from build123d import *

# Parameters (mm, degrees)
F0_R     = 2.7686
F1_DEPTH = 13.208
F2_DEPTH = 10.922
F3_DEPTH = 0.254
F4_DEPTH = 4.953
F5_R     = 2.7686
F6_DEPTH = 6.731
F7_DEPTH = 0.381


with BuildPart() as f1:
    # F0 (on Top) → F1 (new body)
    with BuildSketch(Plane.XY):
        with BuildLine():
            Line((-13.6779, -4.1021), (13.6779, -4.1021))
            ThreePointArc((13.6779, -4.1021), (17.78, 0), (13.6779, 4.1021))
            Line((13.6779, 4.1021), (-13.6779, 4.1021))
            ThreePointArc((-13.6779, 4.1021), (-17.78, 0), (-13.6779, -4.1021))
        make_face()
        with BuildLine():
            ThreePointArc((-13.6779, -3.7211), (-17.399, 0), (-13.6779, 3.7211))
            Line((-13.6779, 3.7211), (13.6779, 3.7211))
            ThreePointArc((13.6779, 3.7211), (17.399, 0), (13.6779, -3.7211))
            Line((13.6779, -3.7211), (-13.6779, -3.7211))
        make_face(mode=Mode.SUBTRACT)
        with BuildLine():
            Line((13.6779, 3.7211), (-13.6779, 3.7211))
            ThreePointArc((-13.6779, 3.7211), (-17.399, 0), (-13.6779, -3.7211))
            Line((-13.6779, -3.7211), (13.6779, -3.7211))
            ThreePointArc((13.6779, -3.7211), (17.399, 0), (13.6779, 3.7211))
        make_face()
        with BuildLine():
            ThreePointArc((-12.875422, 0.0127), (-12.875422, 2.4003), (-10.8077, 3.5941))
            Line((-10.8077, 3.5941), (10.8077, 3.5941))
            ThreePointArc((10.8077, 3.5941), (12.875422, 2.4003), (12.875422, 0.0127))
            Line((12.875422, 0.0127), (11.482276, -2.4003))
            ThreePointArc((11.482276, -2.4003), (10.608354, -3.274222), (9.414554, -3.5941))
            Line((9.414554, -3.5941), (-9.414554, -3.5941))
            ThreePointArc((-9.414554, -3.5941), (-10.608354, -3.274222), (-11.482276, -2.4003))
            Line((-11.482276, -2.4003), (-12.875422, 0.0127))
        make_face(mode=Mode.SUBTRACT)
        with BuildLine():
            Line((10.8077, 3.5941), (-10.8077, 3.5941))
            ThreePointArc((-10.8077, 3.5941), (-12.875422, 2.4003), (-12.875422, 0.0127))
            Line((-12.875422, 0.0127), (-11.482276, -2.4003))
            ThreePointArc((-11.482276, -2.4003), (-10.608354, -3.274222), (-9.414554, -3.5941))
            Line((-9.414554, -3.5941), (9.414554, -3.5941))
            ThreePointArc((9.414554, -3.5941), (10.608354, -3.274222), (11.482276, -2.4003))
            Line((11.482276, -2.4003), (12.875422, 0.0127))
            ThreePointArc((12.875422, 0.0127), (12.875422, 2.4003), (10.8077, 3.5941))
        make_face()
        with BuildLine():
            ThreePointArc((-12.325496, 0.3302), (-12.325496, 2.0828), (-10.8077, 2.9591))
            Line((-10.8077, 2.9591), (10.8077, 2.9591))
            ThreePointArc((10.8077, 2.9591), (12.325496, 2.0828), (12.325496, 0.3302))
            Line((12.325496, 0.3302), (10.93235, -2.0828))
            ThreePointArc((10.93235, -2.0828), (10.290854, -2.724296), (9.414554, -2.9591))
            Line((9.414554, -2.9591), (-9.414554, -2.9591))
            ThreePointArc((-9.414554, -2.9591), (-10.290854, -2.724296), (-10.93235, -2.0828))
            Line((-10.93235, -2.0828), (-12.325496, 0.3302))
        make_face(mode=Mode.SUBTRACT)
        with BuildLine():
            Line((10.8077, 2.9591), (-10.8077, 2.9591))
            ThreePointArc((-10.8077, 2.9591), (-12.325496, 2.0828), (-12.325496, 0.3302))
            Line((-12.325496, 0.3302), (-10.93235, -2.0828))
            ThreePointArc((-10.93235, -2.0828), (-10.290854, -2.724296), (-9.414554, -2.9591))
            Line((-9.414554, -2.9591), (9.414554, -2.9591))
            ThreePointArc((9.414554, -2.9591), (10.290854, -2.724296), (10.93235, -2.0828))
            Line((10.93235, -2.0828), (12.325496, 0.3302))
            ThreePointArc((12.325496, 0.3302), (12.325496, 2.0828), (10.8077, 2.9591))
        make_face()
        with Locations((-8.717981, 0)):
            Circle(F0_R, mode=Mode.SUBTRACT)
        with Locations((8.717981, 0)):
            Circle(F0_R, mode=Mode.SUBTRACT)
    extrude(amount=-F1_DEPTH)

    # F0 (on Top) → F2 (cut)
    with BuildSketch(Plane.XY):
        with BuildLine():
            Line((-13.6779, -4.1021), (13.6779, -4.1021))
            ThreePointArc((13.6779, -4.1021), (17.78, 0), (13.6779, 4.1021))
            Line((13.6779, 4.1021), (-13.6779, 4.1021))
            ThreePointArc((-13.6779, 4.1021), (-17.78, 0), (-13.6779, -4.1021))
        make_face()
        with BuildLine():
            ThreePointArc((-13.6779, -3.7211), (-17.399, 0), (-13.6779, 3.7211))
            Line((-13.6779, 3.7211), (13.6779, 3.7211))
            ThreePointArc((13.6779, 3.7211), (17.399, 0), (13.6779, -3.7211))
            Line((13.6779, -3.7211), (-13.6779, -3.7211))
        make_face(mode=Mode.SUBTRACT)
    extrude(amount=-F2_DEPTH, mode=Mode.SUBTRACT)

    # F0 (on Top) → F3 (cut)
    with BuildSketch(Plane.XY):
        with BuildLine():
            Line((13.6779, 3.7211), (-13.6779, 3.7211))
            ThreePointArc((-13.6779, 3.7211), (-17.399, 0), (-13.6779, -3.7211))
            Line((-13.6779, -3.7211), (13.6779, -3.7211))
            ThreePointArc((13.6779, -3.7211), (17.399, 0), (13.6779, 3.7211))
        make_face()
        with BuildLine():
            ThreePointArc((-12.875422, 0.0127), (-12.875422, 2.4003), (-10.8077, 3.5941))
            Line((-10.8077, 3.5941), (10.8077, 3.5941))
            ThreePointArc((10.8077, 3.5941), (12.875422, 2.4003), (12.875422, 0.0127))
            Line((12.875422, 0.0127), (11.482276, -2.4003))
            ThreePointArc((11.482276, -2.4003), (10.608354, -3.274222), (9.414554, -3.5941))
            Line((9.414554, -3.5941), (-9.414554, -3.5941))
            ThreePointArc((-9.414554, -3.5941), (-10.608354, -3.274222), (-11.482276, -2.4003))
            Line((-11.482276, -2.4003), (-12.875422, 0.0127))
        make_face(mode=Mode.SUBTRACT)
    extrude(amount=-F3_DEPTH, mode=Mode.SUBTRACT)

    # F0 (on Top) → F4 (cut)
    with BuildSketch(Plane.XY):
        with BuildLine():
            Line((10.8077, 2.9591), (-10.8077, 2.9591))
            ThreePointArc((-10.8077, 2.9591), (-12.325496, 2.0828), (-12.325496, 0.3302))
            Line((-12.325496, 0.3302), (-10.93235, -2.0828))
            ThreePointArc((-10.93235, -2.0828), (-10.290854, -2.724296), (-9.414554, -2.9591))
            Line((-9.414554, -2.9591), (9.414554, -2.9591))
            ThreePointArc((9.414554, -2.9591), (10.290854, -2.724296), (10.93235, -2.0828))
            Line((10.93235, -2.0828), (12.325496, 0.3302))
            ThreePointArc((12.325496, 0.3302), (12.325496, 2.0828), (10.8077, 2.9591))
        make_face()
        with Locations((-8.717981, 0)):
            Circle(F0_R, mode=Mode.SUBTRACT)
        with Locations((8.717981, 0)):
            Circle(F0_R, mode=Mode.SUBTRACT)
    extrude(amount=-F4_DEPTH, mode=Mode.SUBTRACT)

    # F5 (on face) → F6 (cut)
    with BuildSketch(Plane(origin=(0, 0, -13.208), x_dir=(1, 0, 0), z_dir=(0, 0, -1))):
        with BuildLine():
            ThreePointArc((-12.325496, -0.3302), (-12.325496, -2.0828), (-10.8077, -2.9591))
            Line((-10.8077, -2.9591), (10.8077, -2.9591))
            ThreePointArc((10.8077, -2.9591), (12.325496, -2.0828), (12.325496, -0.3302))
            Line((12.325496, -0.3302), (10.93235, 2.0828))
            ThreePointArc((10.93235, 2.0828), (10.290854, 2.724296), (9.414554, 2.9591))
            Line((9.414554, 2.9591), (-9.414554, 2.9591))
            ThreePointArc((-9.414554, 2.9591), (-10.290854, 2.724296), (-10.93235, 2.0828))
            Line((-10.93235, 2.0828), (-12.325496, -0.3302))
        make_face()
        with Locations((-8.717981, 0)):
            Circle(F5_R, mode=Mode.SUBTRACT)
        with Locations((8.717981, 0)):
            Circle(F5_R, mode=Mode.SUBTRACT)
    extrude(amount=-F6_DEPTH, mode=Mode.SUBTRACT)

    # F5 (on face) → F7 (cut)
    with BuildSketch(Plane(origin=(0, 0, -13.208), x_dir=(1, 0, 0), z_dir=(0, 0, -1))):
        with BuildLine():
            ThreePointArc((13.6779, -3.7211), (17.399, 0), (13.6779, 3.7211))
            Line((13.6779, 3.7211), (-13.6779, 3.7211))
            ThreePointArc((-13.6779, 3.7211), (-17.399, 0), (-13.6779, -3.7211))
            Line((-13.6779, -3.7211), (13.6779, -3.7211))
        make_face()
        with BuildLine():
            Line((10.8077, -2.9591), (-10.8077, -2.9591))
            ThreePointArc((-10.8077, -2.9591), (-12.325496, -2.0828), (-12.325496, -0.3302))
            Line((-12.325496, -0.3302), (-10.93235, 2.0828))
            ThreePointArc((-10.93235, 2.0828), (-10.290854, 2.724296), (-9.414554, 2.9591))
            Line((-9.414554, 2.9591), (9.414554, 2.9591))
            ThreePointArc((9.414554, 2.9591), (10.290854, 2.724296), (10.93235, 2.0828))
            Line((10.93235, 2.0828), (12.325496, -0.3302))
            ThreePointArc((12.325496, -0.3302), (12.325496, -2.0828), (10.8077, -2.9591))
        make_face(mode=Mode.SUBTRACT)
    extrude(amount=-F7_DEPTH, mode=Mode.SUBTRACT)


solid = f1.part
The listing builds one solid part. Answer for the finished solid, in the listing's coordinates (mm). A direction names the side the tool comes from. Round coordinates to 2 decimals unless told otherwise and drop trailing zeros. Write each loop counter-clockwise with the first axis right and the second up, starting at its lowest first coordinate (ties: lowest second). Pieces come first, ordered by that corner, then holes. Notation, with made-up numbers: (-1.5, 16.5) - (37.5, 16.5) arc R24 cw to (37.5, 37.5) - close; hole circle Ø1 at (76.5, 33). An arc over 180 degrees is marked (long way). Use one line per item in the form item = value. Start each with the question number.
Item 1: A cutting plane is placed at C-C (z = -5.5). Write down the section's boundary in (x, y).
Item 2: Flat-ended cylindrical pins translate along their axes: pin 1 Ø6 at (x, z) = (13, -6) entering from +Y; pin 2 Ø4 at (y, z) = (-1, -3.5) entering from -X; pin 3 Ø3 at (x, z) = (-6.5, -3) entering from -Y; pin 4 Ø7 at (x, z) = (-3.5, -10) entering from +Y. Find the tip coordinate at first contact, or state that the pin passes through.
Item 3: A cutting plane is placed at A-A (z = -9.75). Write down the section's boundary in (x, y), plus the area to 3 significant figures.
Item 4: A cutting plane is placed at B-B (y = 2). Give the number of separate pieces and of enclosed holes in the cut face, plus the area to 3 significant figures.
Item 5: A tool of negligible diameter and unlimited length cuts with its end or side. For faces 1 (the flat face through (0, -3.721, -6)), 2 (the flat face through (-1, 3.2, 0)), 3 (the flat face through (11.62, -0.89, -2.44)), 4 (the flat face through (11.64, -0.86, -9.7)), from which of +Z, -Z, +X, -X, +Y, -Y can it reach the whole face along a straight path? Write none if from no direction.
Item 6: Determine the mould class of faces 5 (the flat face through (0, 2.959, -10)), 6 (the flat face through (0, 4.102, -12)), 7 (the cylindrical face through (-17.78, 0.09, -12.05)), 8 (the flat face through (0, -4.102, -12)) for opening direction Y: +Y half, -Y half, draft (parallel to the pull), parting line (faces both ways), or undercut.
Item 7: A cutting plane is placed at D-D (x = 0). Write down the section's boundary in (y, z).
Item 8: Find the intervals of material crossed by line 1 (X direction, y = 0, z = -5.4); line 2 (Y direction, x = -5.5, z = -4.5); line 3 (Y direction, x = 5.5, z = -5.5), in increasing order. Write a range as [from, to].
The answers:
q1.outline = (-13.68, -3.72) - (13.68, -3.72) arc R3.72 ccw to (13.68, 3.72) - (-13.68, 3.72) arc R3.72 ccw to start; hole circle Ø5.54 at (-8.72, 0); hole circle Ø5.54 at (8.72, 0)
q2.pin_1 = 3.72
q2.pin_2 = -17.4
q2.pin_3 = -3.72
q2.pin_4 = 4.1
q3.outline = (-13.68, -3.72) - (13.68, -3.72) arc R3.72 ccw to (13.68, 3.72) - (-13.68, 3.72) arc R3.72 ccw to start; hole (-12.33, 0.33) - (-10.93, -2.08) arc R1.75 ccw to (-9.41, -2.96) - (9.41, -2.96) arc R1.75 ccw to (10.93, -2.08) - (12.33, 0.33) arc R1.75 ccw to (10.81, 2.96) - (-10.81, 2.96) arc R1.75 ccw to start
q3.area = 108 mm^2
q4.separate_pieces = 3
q4.enclosed_holes = 0
q4.area = 140 mm^2
q5.face_1 = +Z, +X, -X, -Y
q5.face_2 = +Z, +X, -X, +Y, -Y
q5.face_3 = +Z
q5.face_4 = -Z
q6.face_5 = undercut
q6.face_6 = +Y half
q6.face_7 = parting line
q6.face_8 = -Y half
q7.outline = (-4.1, -13.21) - (-3.72, -13.21) - (-3.72, -12.83) - (-2.96, -12.83) - (-2.96, -6.48) - (2.96, -6.48) - (2.96, -12.83) - (3.72, -12.83) - (3.72, -13.21) - (4.1, -13.21) - (4.1, -10.92) - (3.72, -10.92) - (3.72, -0.25) - (3.59, -0.25) - (3.59, 0) - (2.96, 0) - (2.96, -4.95) - (-2.96, -4.95) - (-2.96, 0) - (-3.59, 0) - (-3.59, -0.25) - (-3.72, -0.25) - (-3.72, -10.92) - (-4.1, -10.92) - close
q8.line_1 = [-17.4, -11.49], [-5.95, 5.95], [11.49, 17.4]
q8.line_2 = [-3.72, -2.96], [2.96, 3.72]
q8.line_3 = [-3.72, 3.72]
